```python
from build123d import *

# Parameters (mm, degrees)
ESQUISSE1_R             = 27
BOSS_EXTRU_1_DEPTH      = 38
CONG_1_R                = 3
CONG_2_R                = 3
ESQUISSE2_R             = 17.5
ENL_V_MAT_EXTRU_1_DEPTH = 15
ESQUISSE3_R             = 17.5
ENL_V_MAT_EXTRU_2_DEPTH = 15
ESQUISSE4_R             = 3
ENL_V_MAT_EXTRU_3_DEPTH = 15
CONG_3_R                = 1
CONG_4_R                = 1


with BuildPart() as part:
    # Esquisse1 → Boss.-Extru.1 (new body)
    with BuildSketch(Plane(origin=(0, 0, 0), x_dir=(1, 0, 0), z_dir=(0, 1, 0))):
        Circle(ESQUISSE1_R)
    extrude(amount=BOSS_EXTRU_1_DEPTH)

    # Congé1
    cong_1_edges = [part.edges().sort_by_distance(p)[0] for p in [
        (-27, 38, 0),
    ]]
    fillet(cong_1_edges, radius=CONG_1_R)

    # Congé2
    cong_2_edges = [part.edges().sort_by_distance(p)[0] for p in [
        (-27, 0, 0),
    ]]
    fillet(cong_2_edges, radius=CONG_2_R)

    # Esquisse2 → Enlèv. mat.-Extru.1 (cut)
    with BuildSketch(Plane.XZ):
        Circle(ESQUISSE2_R)
    extrude(amount=-ENL_V_MAT_EXTRU_1_DEPTH, mode=Mode.SUBTRACT)

    # Esquisse3 → Enlèv. mat.-Extru.2 (cut)
    with BuildSketch(Plane(origin=(0, 38, 0), x_dir=(1, 0, 0), z_dir=(0, 1, 0))):
        Circle(ESQUISSE3_R)
    extrude(amount=-ENL_V_MAT_EXTRU_2_DEPTH, mode=Mode.SUBTRACT)

    # Esquisse4 → Enlèv. mat.-Extru.3 (cut)
    with BuildSketch(Plane(origin=(0, 23, 0), x_dir=(1, 0, 0), z_dir=(0, 1, 0))):
        Circle(ESQUISSE4_R)
    extrude(amount=-ENL_V_MAT_EXTRU_3_DEPTH, mode=Mode.SUBTRACT)

    # Congé3
    cong_3_edges = [part.edges().sort_by_distance(p)[0] for p in [
        (-17.5, 38, 0),
    ]]
    fillet(cong_3_edges, radius=CONG_3_R)

    # Congé4
    cong_4_edges = [part.edges().sort_by_distance(p)[0] for p in [
        (-17.5, 0, 0),
    ]]
    fillet(cong_4_edges, radius=CONG_4_R)


solid = part.part
```
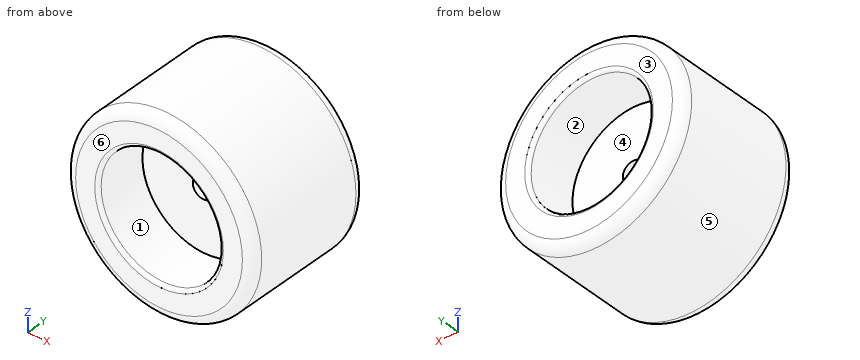
Geometry check sheet. Reference: the model listing, model coordinates, mm. Face numbers are marked on the shaded views. A direction names the side the tool comes from. Give positions to 0.01 mm unless a question says otherwise; leave off trailing zeros. Order: outer loops, then holes, each group sorted by start corner. A loop starts at its lowest first (then second) coordinate and runs counter-clockwise, first axis right, second up.
1. Thickness scan on L1, parallel to Z at x = 0, y = 8; L2, parallel to Z at x = 0, y = 21.25. Record the ranges inside material, lowest first.
2. Access from +Z, -Z, +X, -X, +Y, -Y to the whole of each face (thin tool, end or side, straight path). Record for the marked faces 1, 2 and 3.
3. Release check for a two-part mould opening along Z. For the marked faces 4, 5 and 6 record: pulls with the +Z half, pulls with the -Z half, needs draft (parallel to the pull), parting line crosses it, or undercut.
4. Section check A-A, the plane z = 0. Enter the section's corners in (x, y), and give its area (3 significant figures).
5. Section check C-C, the plane y = 17. Enter the section's corners in (x, z).
6. Gauge pin test, flat ends, axial feed: pin 1 Ø5 at (y, z) = (20, 2.5) entering from -X; pin 2 Ø8 at (x, y) = (17.5, 8.5) entering from +Z; pin 3 Ø12 at (x, z) = (-8, -2) entering from +Y; pin 4 Ø1 at (y, z) = (11, 14.5) entering from -X. Record the tip position at first contact, or that the pin passes through.
7. Section check D-D, the plane y = 10. Enter the section's corners in (x, z), and give its area (3 significant figures).
8. Section check B-B, the plane x = 0. Enter the section's corners in (y, z), and give its area (3 significant figures).
Values follow:
1. L1: z = -27 to -17.5, 17.5 to 27
1. L2: z = -27 to -3, 3 to 27
2. face 1: -Y
2. face 2: +Y
2. face 3: +Z, -Z, +X, -X, +Y
3. face 4: undercut
3. face 5: parting line crosses it
3. face 6: needs draft
4. outline: (-27, 3) arc R3 ccw to (-24, 0) - (-18.5, 0) arc R1 ccw to (-17.5, 1) - (-17.5, 15) - (-3, 15) - (-3, 23) - (-17.5, 23) - (-17.5, 37) arc R1 ccw to (-18.5, 38) - (-24, 38) arc R3 ccw to (-27, 35) - close; (3, 15) - (17.5, 15) - (17.5, 1) arc R1 ccw to (18.5, 0) - (24, 0) arc R3 ccw to (27, 3) - (27, 35) arc R3 ccw to (24, 38) - (18.5, 38) arc R1 ccw to (17.5, 37) - (17.5, 23) - (3, 23) - close
4. area: 945 mm2
5. outline: circle Ø54 at (0, 0); hole circle Ø6 at (0, 0)
6. pin 1: stops at x = -27
6. pin 2: stops at z = 23.38
6. pin 3: stops at y = 23
6. pin 4: stops at x = -23.09
7. outline: circle Ø54 at (0, 0); hole circle Ø35 at (0, 0)
7. area: 1,330 mm2
8. outline: (0, -24) arc R3 ccw to (3, -27) - (35, -27) arc R3 ccw to (38, -24) - (38, -18.5) arc R1 ccw to (37, -17.5) - (23, -17.5) - (23, -3) - (15, -3) - (15, -17.5) - (1, -17.5) arc R1 ccw to (0, -18.5) - close; (0, 18.5) arc R1 ccw to (1, 17.5) - (15, 17.5) - (15, 3) - (23, 3) - (23, 17.5) - (37, 17.5) arc R1 ccw to (38, 18.5) - (38, 24) arc R3 ccw to (35, 27) - (3, 27) arc R3 ccw to (0, 24) - close
8. area: 945 mm2
